Autodesk Inventor part; units mm, degrees
ref_plane "YZ Plane" through (0, 0, 0) normal (1, 0, 0) x (0, 1, 0)
ref_plane "XZ Plane" through (0, 0, 0) normal (0, 1, 0) x (-1, 0, 0)
ref_plane "XY Plane" through (0, 0, 0) normal (0, 0, 1) x (1, 0, 0)
sketch "スケッチ1" plane through (0, 0, 0) normal (0, 1, 0) x (-1, 0, 0)
  line L0 (0, -149.7212) -> (0, 30.7869)
  line L1 (-30.7969, 0) -> (149.7814, 0)
  arc A0 (3.2253, -195.9735) -> (195.977, -3) centre (0, 0) ccw
  arc A1 (3.2253, -203.9745) -> (203.9779, -3) centre (0, 0) ccw
  line L2 (195, 3) -> (195, 5)
  line L3 (195, 5) -> (205, 5)
  line L4 (205, 5) -> (205, 3)
  line L5 (205, 3) -> (195, 3)
  line L6 (203.9779, -3) -> (195.977, -3)
  line L7 (-3, -195) -> (-5, -195)
  line L8 (-5, -195) -> (-5, -205)
  line L9 (-5, -205) -> (-3, -205)
  line L10 (-3, -205) -> (-3, -195)
  line L11 (3.2253, -195.9735) -> (3.2253, -203.9745)
  dimension "d0" = 204
  dimension "d1" = 196
  dimension "d2" = 205
  dimension "d3" = 195
  dimension "d4" = 5
  dimension "d5" = 3
  dimension "d6" = 195
  dimension "d7" = 205
  dimension "d8" = 5
  dimension "d9" = 3
  dimension "d14" = 3
  dimension "d15" = 3.2253
extrude "押し出し1" add sketch "スケッチ1" along normal mid plane 8 contours A0 L6 A1 L11
revolve "回転1" add sketch "スケッチ1" angle 360 about axis through (0, 0, 0) along (-1, 0, 0) contours L2 L3 L4 L5
revolve "回転2" add sketch "スケッチ1" angle 360 about axis through (0, 0, 0) along (0, 0, 1) contours L10 L9 L8 L7
equation "\"d0\" = FrameRadius + 0.5 * FrameThickness"
equation "\"d1\" = FrameRadius - 0.5 * FrameThickness"
equation "\"d2\" = FrameRadius + 0.5 * BossLength"
equation "\"d3\" = FrameRadius - 0.5 * BossLength"
equation "\"d4\" = BossRadius"
equation "\"d5\" = BossHoleRadius"
equation "\"d6\" = FrameRadius - 0.5 * BossLength"
equation "\"d7\" = FrameRadius + 0.5 * BossLength"
equation "\"d8\" = BossRadius"
equation "\"d9\" = BossHoleRadius"
equation "\"d14\" = BossHoleRadius"
equation "\"d10\" = FrameThickness"
equation "\"FrameThickness\" = 8"
equation "\"BossRadius\" = 5"
equation "\"BossHoleRadius\" = 3"
properties part number "ArcFrameRa"
Model file for the job. Use its own axes, mm. A direction names the side the tool comes from. Give positions to 0.01 mm unless a question says otherwise; leave off trailing zeros. Loops run counter-clockwise (first coordinate to the right, second up) from the corner with the lowest first, then second, coordinate; pieces in that order, holes last. Notation, with made-up numbers: (21.25, 84) -> (60.25, 84) arc R28 ccw to (60.25, 118) -> close; hole circle Ø9 at (79.5, -32.75). An arc over 180 degrees is marked (long way). Use a Markdown table: item, result. Add a question column.
(1) Slice it at C-C on x = -91. List the corners of the cut face in (y, z).
(2) Mould opens along Y. For faces 3 (the flat face through (-140, 4, -140)), 4 (the cylindrical face through (-3, 0, -200)), 5 (the flat face through (3.3, 0.1, -195)) say: +Y half, -Y half, draft (parallel to the pull), parting line (faces both ways), or undercut.
(3) Tool access for faces 1 (the cylindrical face through (-200, 0, -3)), 2 (the flat face through (-195, 0.1, 3.3)): list every direction of +Z, -Z, +X, -X, +Y, -Y with a clear straight run to the whole face (end or side of a thin tool).
(4) Wall check: line 1 along Y through (x, z) = (0, -200.75); line 2 along X through (y, z) = (3.5, -141); line 3 along Z through (x, y) = (-138, -0.25). Give the ranges that are in metal, low to high.
(5) Slice it at D-D on z = -40. List the corners of the cut face in (x, y), and give its area (3 significant figures).
(6) Drop flat-ended pins along their axis: pin 1 Ø1.5 at (y, z) = (1, -35.5) entering from +X; pin 2 Ø2 at (x, y) = (-63.5, -3) entering from +Z; pin 3 Ø4 at (y, z) = (0.5, -100) entering from +X. Give the stop position or say it passes through.
(7) Slice it at B-B on y = 0. List the corners of the cut face in (x, z).
(8) Slice it at A-A on z = 0. List the corners of the cut face in (x, y).
Filled sheet:
| question | item | result |
|---|---|---|
| 1 | outline | (-4, -182.58) -> (4, -182.58) -> (4, -173.59) -> (-4, -173.59) -> close |
| 2 | face 3 | +Y half |
| 2 | face 4 | undercut |
| 2 | face 5 | draft |
| 3 | face 1 | +X, -X |
| 3 | face 2 | +Z, +X, +Y, -Y |
| 4 | line 1 | -5 to -3, 3 to 5 |
| 4 | line 2 | -147.43 to -136.14 |
| 4 | line 3 | -150.24 to -139.18 |
| 5 | outline | (-200.04, -4) -> (-191.87, -4) -> (-191.87, 4) -> (-200.04, 4) -> close |
| 5 | area | 65.3 mm2 |
| 6 | pin 1 | x = -192.62 |
| 6 | pin 2 | z = -185.08 |
| 6 | pin 3 | x = -167.37 |
| 7 | outline | (-205, -5) -> (-203.94, -5) arc R204 ccw to (-5, -203.94) -> (-5, -205) -> (-3, -205) -> (-3, -195) -> (-5, -195) -> (-5, -195.94) arc R196 cw to (-195.94, -5) -> (-195, -5) -> (-195, -3) -> (-205, -3) -> close; (-205, 3) -> (-195, 3) -> (-195, 5) -> (-205, 5) -> close; (3, -205) -> (5, -205) -> (5, -195) -> (3, -195) -> close |
| 8 | outline | (-205, -5) -> (-195, -5) -> (-195, -3) -> (-205, -3) -> close; (-205, 3) -> (-195, 3) -> (-195, 5) -> (-205, 5) -> close |
